from build123d import *

# Parameters (mm, degrees)
SKETCH1_W           = 85
SKETCH1_H           = 56
SKETCH1_R           = 1.375
BOSS_EXTRUDE1_DEPTH = 3
FILLET1_R           = 3
SKETCH3_R           = 3
SKETCH3_R_2         = 1.375
BOSS_EXTRUDE3_DEPTH = 3
SKETCH5_W           = 5
SKETCH5_H           = 5
SKETCH5_R           = 1.25
BOSS_EXTRUDE4_DEPTH = 2
FILLET2_R           = 2.5
SKETCH6_W           = 5
SKETCH6_H           = 5
SKETCH6_R           = 1.25
BOSS_EXTRUDE5_DEPTH = 2
FILLET3_R           = 2.5
SKETCH8_W           = 5
SKETCH8_H           = 5
SKETCH8_R           = 1.25
BOSS_EXTRUDE7_DEPTH = 2
FILLET5_R           = 2.5


with BuildPart() as part:
    # Sketch1 → Boss-Extrude1 (new body)
    with BuildSketch(Plane(origin=(0, 0, 0), x_dir=(1, 0, 0), z_dir=(0, 1, 0))):
        with Locations((42.5, 28)):
            Rectangle(SKETCH1_W, SKETCH1_H)
        with Locations(Location((3.5, 52.5, 0), (0, 0, 270))):
            Circle(SKETCH1_R, mode=Mode.SUBTRACT)
        with Locations(Location((61.5, 52.5, 0), (0, 0, 270))):
            Circle(SKETCH1_R, mode=Mode.SUBTRACT)
        with Locations(Location((3.5, 3.5, 0), (0, 0, 270))):
            Circle(SKETCH1_R, mode=Mode.SUBTRACT)
        with Locations(Location((61.5, 3.5, 0), (0, 0, 270))):
            Circle(SKETCH1_R, mode=Mode.SUBTRACT)
    extrude(amount=BOSS_EXTRUDE1_DEPTH)

    # Fillet1
    fillet1_edges = [part.edges().sort_by_distance(p)[0] for p in [
        (0, 1.5, -56),
        (85, 1.5, -56),
        (85, 1.5, 0),
        (0, 1.5, 0),
    ]]
    fillet(fillet1_edges, radius=FILLET1_R)

    # Sketch3 → Boss-Extrude3 (add)
    # profile 1 of 4: a face of its own
    with BuildSketch(Plane(origin=(0, 3, 0), x_dir=(1, 0, 0), z_dir=(0, 1, 0))):
        with Locations(Location((3.5, 52.5, 0), (0, 0, 270))):
            Circle(SKETCH3_R)
        with Locations(Location((3.5, 52.5, 0), (0, 0, 270))):
            Circle(SKETCH3_R_2, mode=Mode.SUBTRACT)
    # profile 2 of 4: a face of its own
    with BuildSketch(Plane(origin=(0, 3, 0), x_dir=(1, 0, 0), z_dir=(0, 1, 0))):
        with Locations(Location((61.5, 52.5, 0), (0, 0, 270))):
            Circle(SKETCH3_R)
        with Locations(Location((61.5, 52.5, 0), (0, 0, 270))):
            Circle(SKETCH3_R_2, mode=Mode.SUBTRACT)
    # profile 3 of 4: a face of its own
    with BuildSketch(Plane(origin=(0, 3, 0), x_dir=(1, 0, 0), z_dir=(0, 1, 0))):
        with Locations(Location((3.5, 3.5, 0), (0, 0, 270))):
            Circle(SKETCH3_R)
        with Locations(Location((3.5, 3.5, 0), (0, 0, 270))):
            Circle(SKETCH3_R_2, mode=Mode.SUBTRACT)
    # profile 4 of 4: a face of its own
    with BuildSketch(Plane(origin=(0, 3, 0), x_dir=(1, 0, 0), z_dir=(0, 1, 0))):
        with Locations(Location((61.5, 3.5, 0), (0, 0, 270))):
            Circle(SKETCH3_R)
        with Locations(Location((61.5, 3.5, 0), (0, 0, 270))):
            Circle(SKETCH3_R_2, mode=Mode.SUBTRACT)
    extrude(amount=BOSS_EXTRUDE3_DEPTH)

    # Sketch5 → Boss-Extrude4 (add)
    with BuildSketch(Plane.XZ):
        with Locations((29, 2.5)):
            Rectangle(SKETCH5_W, SKETCH5_H)
        with Locations(Location((29, 2.5, 0), (0, 0, 270))):
            Circle(SKETCH5_R, mode=Mode.SUBTRACT)
    extrude(amount=-BOSS_EXTRUDE4_DEPTH)

    # Fillet2
    fillet2_edges = [part.edges().sort_by_distance(p)[0] for p in [
        (26.5, 1, 5),
        (31.5, 1, 5),
    ]]
    fillet(fillet2_edges, radius=FILLET2_R - 0.0001)  # a hair under: the kernel refuses the full size

    # Sketch6 → Boss-Extrude5 (add)
    with BuildSketch(Plane.XZ):
        with Locations((29, -58.5)):
            Rectangle(SKETCH6_W, SKETCH6_H)
        with Locations(Location((29, -58.5, 0), (0, 0, 270))):
            Circle(SKETCH6_R, mode=Mode.SUBTRACT)
    extrude(amount=-BOSS_EXTRUDE5_DEPTH)

    # Fillet3
    fillet3_edges = [part.edges().sort_by_distance(p)[0] for p in [
        (31.5, 1, -61),
        (26.5, 1, -61),
    ]]
    fillet(fillet3_edges, radius=FILLET3_R - 0.0001)  # a hair under: the kernel refuses the full size

    # Sketch8 → Boss-Extrude7 (add)
    with BuildSketch(Plane.XZ):
        with Locations((87.5, -28)):
            Rectangle(SKETCH8_W, SKETCH8_H)
        with Locations(Location((87.5, -28, 0), (0, 0, 270))):
            Circle(SKETCH8_R, mode=Mode.SUBTRACT)
    extrude(amount=-BOSS_EXTRUDE7_DEPTH)

    # Fillet5
    fillet5_edges = [part.edges().sort_by_distance(p)[0] for p in [
        (90, 1, -30.5),
        (90, 1, -25.5),
    ]]
    fillet(fillet5_edges, radius=FILLET5_R - 0.0001)  # a hair under: the kernel refuses the full size


solid = part.part
The listing builds one solid part. Answer for the finished solid, in the listing's coordinates (mm). A direction names the side the tool comes from. Coordinates: 2 decimals unless noted, no trailing zeros. Loops run counter-clockwise (first coordinate to the right, second up) from the corner with the lowest first, then second, coordinate; pieces in that order, holes last. Notation, with made-up numbers: (77.5, -6.75) -> (92.5, -6.75) arc R36 cw to (92.5, 30.25) -> close; hole circle Ø4 at (-38, -2.5). An arc over 180 degrees is marked (long way). Answer in a Markdown table with one row per item. Add a question column.
1. The part is cut by section A-A, the plane y = 5.1. Write down the section's boundary in (x, z) (3 decimals), then the cut area to 3 significant figures.
2. For faces 1 (the flat face through (26.5, 1, 1)), 2 (the flat face through (86, 1, -30.5)), 3 (the flat face through (26.5, 1, -57)), 4 (the flat face through (42, 3, -28)), determine the directions among +Z, -Z, +X, -X, +Y, -Y from which every point of the face is accessible in a straight line to the end or side of a thin tool.
3. Consider line 1 (X direction, y = 4, z = -3.5) (3 decimals); line 2 (X direction, y = 1.25, z = 2.5); line 3 (Y direction, x = 15, z = -48). Determine where each line is inside the solid, lowest interval first. Write a range as [from, to].
4. The part is cut by section B-B, the plane x = 57.5. Write down the section's boundary in (y, z).
5. Flat-ended cylindrical pins translate along their axes: P1, Ø2, axis at y = 1.5, z = -57.5, coming from the -X side; P2, Ø5.5, axis at x = 30, z = -59, coming from the +Y side; P3, Ø2.5, axis at y = 1.5, z = -16, coming from the +X side; P4, Ø2, axis at x = 87.5, z = -28, coming from the -Y side. Find the tip coordinate at first contact, or state that the pin passes through.
6. The part is cut by section C-C, the plane z = -32. Write down the section's boundary in (x, y).
7. Determine the mould class of faces 5 (the cylindrical face through (64.474, 4.479, -3.891)), 6 (the flat face through (86, 1, -25.5)), 7 (the cylindrical face through (84.1, 1.52, -55.14)) for opening direction X: +X half, -X half, draft (parallel to the pull), parting line (faces both ways), or undercut.
Answer below:
| question | item | result |
|---|---|---|
| 1 | outline | circle Ø6 at (3.5, -52.5); circle Ø6 at (3.5, -3.5); circle Ø6 at (61.5, -52.5); circle Ø6 at (61.5, -3.5); hole circle Ø2.75 at (3.5, -52.5); hole circle Ø2.75 at (3.5, -3.5); hole circle Ø2.75 at (61.5, -52.5); hole circle Ø2.75 at (61.5, -3.5) |
| 1 | area | 89.3 mm2 |
| 2 | face 1 | +Z, -X, +Y, -Y |
| 2 | face 2 | -Z, +X, +Y, -Y |
| 2 | face 3 | -Z, -X, +Y, -Y |
| 2 | face 4 | +Y |
| 3 | line 1 | [0.5, 2.125], [4.875, 6.5], [58.5, 60.125], [62.875, 64.5] |
| 3 | line 2 | [26.5, 27.75], [30.25, 31.5] |
| 3 | line 3 | [0, 3] |
| 4 | outline | (0, -56) -> (3, -56) -> (3, 0) -> (0, 0) -> close |
| 5 | P1 | x = 26.5 |
| 5 | P2 | y = 2 |
| 5 | P3 | x = 85 |
| 5 | P4 | through |
| 6 | outline | (0, 0) -> (85, 0) -> (85, 3) -> (0, 3) -> close |
| 7 | face 5 | undercut |
| 7 | face 6 | draft |
| 7 | face 7 | +X half |
